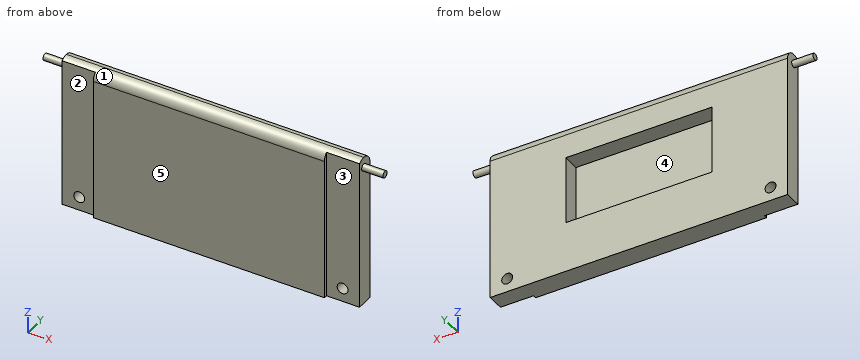
from build123d import *

# Parameters (mm, degrees)
EXTRUDE_1_DEPTH     = 45
SKETCH_2_W          = 43
SKETCH_2_H          = 20
CUT_EXTRUDE_2_DEPTH = 5
FILLET_2_R          = 3
EXTRUDE_START       = -43.75
SKETCH_4_R          = 1
EXTRUDE_2_DEPTH     = 50
CUT_EXTRUDE_3_REACH = 69.454
SKETCH_5_R          = 1.6


with BuildPart() as part:
    # 草图1 → 凸台-拉伸1 (new body)
    with BuildSketch(Plane.XY):
        Polygon((34, -2.5), (43.75, -2.5), (43.75, 2.5), (-43.75, 2.5), (-43.75, -2.5), (-34, -2.5), (-34, -3.5), (34, -3.5), align=None)
    extrude(amount=EXTRUDE_1_DEPTH)

    # 草图2 → 切除-拉伸2 (cut)
    with BuildSketch(Plane(origin=(0, 2.5, 0), x_dir=(1, 0, 0), z_dir=(0, 1, 0))):
        with Locations((0, -25)):
            Rectangle(SKETCH_2_W, SKETCH_2_H)
    extrude(amount=-CUT_EXTRUDE_2_DEPTH, mode=Mode.SUBTRACT)

    # 圆角2
    fillet_2_edges = [part.edges().sort_by_distance(p)[0] for p in [
        (0, -3.5, 45),
        (0, 2.5, 45),
    ]]
    fillet(fillet_2_edges, radius=FILLET_2_R - 0.0001)  # a hair under: the kernel refuses the full size

    # 草图4 → 凸台-拉伸2 (add, symmetric)
    with BuildSketch(Plane.ZY.offset(43.75).offset(EXTRUDE_START)):
        with Locations(Location((42, -0.5, 0), (0, 0, 180))):
            Circle(SKETCH_4_R)
    extrude(amount=EXTRUDE_2_DEPTH, both=True)

    # 草图5 → 切除-拉伸3 (cut, up to next)
    with BuildSketch(Plane.XZ.offset(2.5), mode=Mode.PRIVATE) as cut_extrude_3_sk1:
        with Locations(Location((-38.75, 4, 0), (0, 0, 270))):
            Circle(SKETCH_5_R)
    cut_extrude_3_tool1 = extrude(cut_extrude_3_sk1.sketch, amount=-CUT_EXTRUDE_3_REACH, mode=Mode.PRIVATE) & part.part
    cut_extrude_3 = cut_extrude_3_tool1.solids().sort_by_distance((-38.75, -2.5, 4))[0]
    add(cut_extrude_3, mode=Mode.SUBTRACT)

    # 镜向1: 切除-拉伸3 across plane
    add(cut_extrude_3.mirror(Plane(origin=(0, 0, 0), x_dir=(0, 0, 1), z_dir=(1, 0, 0))), mode=Mode.SUBTRACT)


solid = part.part
Geometry: final body of the model. Coordinates: model frame, mm. Face numbers are marked on the shaded views. A direction names the side the tool comes from. Give positions to 0.01 mm unless a question says otherwise; leave off trailing zeros. Order: outer loops, then holes, each group sorted by start corner. A loop starts at its lowest first (then second) coordinate and runs counter-clockwise, first axis right, second up. Notation, with made-up numbers: (52.25, -13.5) -> (105.25, -13.5) arc R23 ccw to (105.25, 12.5) -> close; hole circle Ø4 at (3, 12). An arc over 180 degrees is marked (long way). Put each result on its own line as item: value.
Q1. Pin query (flat end, axial travel): pin 1 (2.5 mm diameter, centred on y = -1, z = 23, fed in from +X); pin 2 (3 mm diameter, centred on x = -40, z = 30, fed in from -Y); pin 3 (2.5 mm diameter, centred on x = 38.75, z = 4, fed in from +Y); pin 4 (2 mm diameter, centred on x = 3.5, y = -2.5, fed in from +Z). Return the tip coordinate at first contact, or that it passes through.
Here are the results:
pin 1: stops at x = 43.75
pin 2: stops at y = -2.5
pin 3: passes through
pin 4: stops at z = 44.83
Q2. Section B-B, the plane z = 4. Return loops of the section in (x, y).
Here are the results:
outline: (-43.75, -2.5) -> (-40.35, -2.5) -> (-40.35, 2.5) -> (-43.75, 2.5) -> close; (-37.15, -2.5) -> (-34, -2.5) -> (-34, -3.5) -> (34, -3.5) -> (34, -2.5) -> (37.15, -2.5) -> (37.15, 2.5) -> (-37.15, 2.5) -> close; (40.35, -2.5) -> (43.75, -2.5) -> (43.75, 2.5) -> (40.35, 2.5) -> close
Q3. Section C-C, the plane z = 11.5. Return loops of the section in (x, y).
Here are the results:
outline: (-43.75, -2.5) -> (-34, -2.5) -> (-34, -3.5) -> (34, -3.5) -> (34, -2.5) -> (43.75, -2.5) -> (43.75, 2.5) -> (-43.75, 2.5) -> close
Q4. Material intervals for L1, parallel to X at y = 1.4, z = 4; L2, parallel to X at y = 1.5, z = 27.5; L3, parallel to X at y = -2.75, z = 4, sorted ascending.
Here are the results:
L1: x = -43.75 to -40.35, -37.15 to 37.15, 40.35 to 43.75
L2: x = -43.75 to -21.5, 21.5 to 43.75
L3: x = -34 to 34
Q5. Reachability of the marked faces 1, 2 and 3 from +Z, -Z, +X, -X, +Y, -Y: full face, straight path, thin tool, end or side. Return the list, or none.
Here are the results:
face 1: +Z, +X, -X, -Y
face 2: +Z, -Z, -X, -Y
face 3: +Z, -Z, +X, -Y
Q6. Draft query along X for the marked faces 4 and 5. Return one class per face: released by +X, released by -X, zero draft, split by the parting line, or undercut.
Here are the results:
face 4: undercut
face 5: zero draft
